Check sheet for the modelled part. Datum: model origin and axes. Units: mm. A direction names the side the tool comes from. Round coordinates to 2 decimals unless told otherwise and drop trailing zeros. Loops run counter-clockwise (first coordinate to the right, second up) from the corner with the lowest first, then second, coordinate; pieces in that order, holes last. Notation, with made-up numbers: (2.25, -26.75) - (42.25, -26.75) arc R17 cw to (42.25, 0.25) - close; hole circle Ø10 at (32.25, -4.5). An arc over 180 degrees is marked (long way). Answer in a Markdown table with one row per item. Add a question column.
(1) Thickness scan on line 1 along Y through (x, z) = (1.5, -3.25); line 2 along Z through (x, y) = (1, 4); line 3 along Z through (x, y) = (1, 11.5). Record the ranges inside material, lowest first.
(2) Cross-section at B-B on y = 7.25. Enter the section's corners in (x, z), then the cut area to 3 significant figures.
(3) Access from +Z, -Z, +X, -X, +Y, -Y to the whole of each face (thin tool, end or side, straight path). Record for faces 1 (the cylindrical face through (2.385, 8.01, -0.751)), 2 (the cylindrical face through (-0.54, 3.23, 2.44)), 3 (the conical face through (0.556, 4.93, 0.936)).
(4) Gauge pin test, flat ends, axial feed: pin 1 (2.5 mm diameter, centred on x = -0.5, z = 2, fed in from +Y); pin 2 (1.5 mm diameter, centred on x = -0.5, y = 2.5, fed in from +Z); pin 3 (1 mm diameter, centred on x = 2, y = 10.5, fed in from -Z). Record the tip position at first contact, or that the pin passes through.
(5) Mould release check, pull along X, two halves, no side actions. Record for faces 4 (the flat face through (1, 1.5, -3)), 5 (the conical face through (0.53, 4.93, -0.95)), 6 (the cylindrical face through (-0.99, 0.74, -4.44)): +X half, -X half, draft (parallel to the pull), parting line (faces both ways), or undercut.
(6) Cross-section at A-A on y = 2.25. Enter the section's corners in (x, z).
from build123d import *

# Parameters (mm, degrees)
SKETCH1_R           = 2.5
BOSS_EXTRUDE1_DEPTH = 12
SKETCH6_R           = 4.55
BOSS_EXTRUDE3_DEPTH = 1.5
SKETCH2_R           = 1
CUT_EXTRUDE1_DEPTH  = 10
DRAFT1_ANGLE        = 1
BOSS_EXTRUDE2_DEPTH = 10
FILLET1_R           = 0.5


with BuildPart() as part:
    # Sketch1 → Boss-Extrude1 (new body)
    with BuildSketch(Plane(origin=(0, 0, 0), x_dir=(1, 0, 0), z_dir=(0, 1, 0))):
        Circle(SKETCH1_R)
    extrude(amount=BOSS_EXTRUDE1_DEPTH)

    # Sketch6 → Boss-Extrude3 (add)
    with BuildSketch(Plane.XZ):
        Circle(SKETCH6_R)
    extrude(amount=-BOSS_EXTRUDE3_DEPTH)

    # Sketch8 → Revolve1 (revolve)
    with BuildSketch(Plane.XY):
        with BuildLine():
            Line((2.5, 6.353553391), (3.426776695, 5.426776695))
            ThreePointArc((3.426776695, 5.426776695), (3.480969883, 5.154329142), (3.25, 5))
            Line((3.25, 5), (2.5, 5))
            Line((2.5, 5), (2.5, 6.353553391))
        make_face()
    revolve(axis=Axis((0, 0, 0), (0, 1, 0)))

    # Sketch2 → Cut-Extrude1 (cut)
    with BuildSketch(Plane.XZ):
        Circle(SKETCH2_R)
    extrude(amount=-CUT_EXTRUDE1_DEPTH, mode=Mode.SUBTRACT)

    # Draft1
    draft1_faces = [part.faces().sort_by_distance(p)[0] for p in [
        (-1, 5, 0),
    ]]
    draft(draft1_faces, Plane(origin=(0, 10, 0), x_dir=(0, 0, -1), z_dir=(0, -1, 0)), DRAFT1_ANGLE)

    # Sketch7 → Cut-Revolve3 (revolve, cut)
    with BuildSketch(Plane.XY):
        with BuildLine():
            Line((2.5, 9.5), (3.080651327, 9.5))
            Line((3.080651327, 9.5), (3.080651327, 12.580651327))
            Line((3.080651327, 12.580651327), (0, 12.580651327))
            Line((0, 12.580651327), (0, 12))
            ThreePointArc((0, 12), (1.767766953, 11.267766953), (2.5, 9.5))
        make_face()
    revolve(axis=Axis((0, 9.5, 0), (0, 1, 0)), mode=Mode.SUBTRACT)

    # Sketch3 → Boss-Extrude2 (add)
    with BuildSketch(Plane.XZ.offset(-10)):
        with BuildLine():
            Line((1.151036246, 0.233847786), (0.746, 0))
            Line((0.746, 0), (1.151036246, -0.233847786))
            ThreePointArc((1.151036246, -0.233847786), (1.174550649, 0), (1.151036246, 0.233847786))
        make_face()
        with BuildLine():
            Line((-0.373, -1.113750523), (-0.373, -0.646054951))
            Line((-0.373, -0.646054951), (-0.778036246, -0.879902737))
            ThreePointArc((-0.778036246, -0.879902737), (-0.587275325, -1.0171907), (-0.373, -1.113750523))
        make_face()
        with BuildLine():
            Line((-0.778036246, 0.879902737), (-0.373, 0.646054951))
            Line((-0.373, 0.646054951), (-0.373, 1.113750523))
            ThreePointArc((-0.373, 1.113750523), (-0.587275325, 1.0171907), (-0.778036246, 0.879902737))
        make_face()
    extrude(amount=BOSS_EXTRUDE2_DEPTH)

    # Sketch4 → Cut-Revolve1 (revolve, cut)
    with BuildSketch(Plane.XY):
        Polygon((1.174550649, 0), (0.746, 0.510726776), (0, 0.510726776), (0, 0), align=None)
    revolve(axis=Axis((0, 0.510726776, 0), (0, -1, 0)), mode=Mode.SUBTRACT)

    # Fillet1
    fillet1_edges = [part.edges().sort_by_distance(p)[0] for p in [
        (-2.5, 5, 0),
        (-2.5, 6.353553391, 0),
        (-2.5, 1.5, 0),
    ]]
    fillet(fillet1_edges, radius=FILLET1_R)


solid = part.part
Answers:
| question | item | result |
|---|---|---|
| 1 | line 1 | y = 0 to 1.5 |
| 1 | line 2 | z = -2.29 to -0.47, -0.15 to 0.15, 0.47 to 2.29 |
| 1 | line 3 | z = -1.12 to 1.12 |
| 2 | outline | circle Ø5 at (0, 0); hole (-0.66, -0.81) - (-0.37, -0.65) - (-0.37, -0.98) arc R1.05 ccw to (1.03, -0.17) - (0.75, 0) - (1.03, 0.17) arc R1.05 ccw to (-0.37, 0.98) - (-0.37, 0.65) - (-0.66, 0.81) arc R1.05 ccw to start |
| 2 | area | 16.3 mm^2 |
| 3 | face 1 | +Y |
| 3 | face 2 | none |
| 3 | face 3 | -Y |
| 4 | pin 1 | stops at y = 11.86 |
| 4 | pin 2 | stops at z = 2.53 |
| 4 | pin 3 | stops at z = -1.8 |
| 5 | face 4 | draft |
| 5 | face 5 | undercut |
| 5 | face 6 | parting line |
| 6 | outline | circle Ø5 at (0, 0); hole (-0.74, -0.86) - (-0.37, -0.65) - (-0.37, -1.07) arc R1.14 ccw to (1.12, -0.21) - (0.75, 0) - (1.12, 0.21) arc R1.14 ccw to (-0.37, 1.07) - (-0.37, 0.65) - (-0.74, 0.86) arc R1.14 ccw to start |
